```python
from build123d import *

# Parameters (mm, degrees)
CROQUIS1_R              = 9.25
SALIENTE_EXTRUIR1_DEPTH = 9.75
REDONDEO4_R             = 3
REDONDEO5_R             = 2
REDONDEO6_R             = 5


with BuildPart() as part:
    # Croquis1 → Saliente-Extruir1 (new, symmetric)
    with BuildSketch(Plane.XY):
        with BuildLine():
            Line((16.461713879, 5.938179534), (18.205490224, 1.104114294))
            ThreePointArc((18.205490224, 1.104114294), (19.855946903, -1.814596224), (22.378427867, -4.023661212))
            ThreePointArc((22.378427867, -4.023661212), (30.919049272, -8.178302275), (40.105510362, -10.589150466))
            ThreePointArc((40.105510362, -10.589150466), (44.326282594, -12.959198031), (46, -17.50130258))
            Line((46, -17.50130258), (46, -18.509558121))
            Line((46, -18.509558121), (46, -43))
            Line((46, -43), (15, -43))
            Line((15, -43), (12, -18))
            Line((12, -18), (-12, -18))
            Line((-12, -18), (-15, -43))
            Line((-15, -43), (-46, -43))
            Line((-46, -43), (-46, -18.509558121))
            Line((-46, -18.509558121), (-46, -17.50130258))
            ThreePointArc((-46, -17.50130258), (-44.326282594, -12.959198031), (-40.105510362, -10.589150466))
            ThreePointArc((-40.105510362, -10.589150466), (-30.919049272, -8.178302275), (-22.378427867, -4.023661212))
            ThreePointArc((-22.378427867, -4.023661212), (-19.855946903, -1.814596224), (-18.205490224, 1.104114294))
            Line((-18.205490224, 1.104114294), (-16.461713879, 5.938179534))
            ThreePointArc((-16.461713879, 5.938179534), (0, 17.5), (16.461713879, 5.938179534))
        make_face()
        Circle(CROQUIS1_R, mode=Mode.SUBTRACT)
    extrude(amount=SALIENTE_EXTRUIR1_DEPTH, both=True)

    # Redondeo4
    redondeo4_edges = [part.edges().sort_by_distance(p)[0] for p in [
        (12, -18, 0),
        (-12, -18, 0),
    ]]
    fillet(redondeo4_edges, radius=REDONDEO4_R)

    # Redondeo5
    redondeo5_edges = [part.edges().sort_by_distance(p)[0] for p in [
        (-19.855946903, -1.814596224, 9.75),
        (-30.919049272, -8.178302275, 9.75),
        (17.333602052, 3.521146914, -9.75),
        (-44.326282594, -12.959198031, 9.75),
        (19.855946903, -1.814596224, -9.75),
        (30.919049272, -8.178302275, -9.75),
        (44.326282594, -12.959198031, -9.75),
        (46, -30.25065129, -9.75),
        (-46, -30.25065129, 9.75),
        (-13.65855386, -31.821282169, -9.75),
        (-46, -30.25065129, -9.75),
        (-44.326282594, -12.959198031, -9.75),
        (-30.919049272, -8.178302275, -9.75),
        (-19.855946903, -1.814596224, -9.75),
        (-17.333602052, 3.521146914, -9.75),
        (0, 17.5, -9.75),
        (-13.65855386, -31.821282169, 9.75),
        (0, 17.5, 9.75),
        (46, -30.25065129, 9.75),
        (44.326282594, -12.959198031, 9.75),
        (30.919049272, -8.178302275, 9.75),
        (19.855946903, -1.814596224, 9.75),
        (13.65855386, -31.821282169, -9.75),
        (13.65855386, -31.821282169, 9.75),
        (0, -18, -9.75),
        (17.333602052, 3.521146914, 9.75),
        (0, -18, 9.75),
        (11.329418316, -18.755862417, -9.75),
        (11.329418316, -18.755862417, 9.75),
        (-11.329418316, -18.755862417, -9.75),
        (-11.329418316, -18.755862417, 9.75),
        (-17.333602052, 3.521146914, 9.75),
    ]]
    fillet(redondeo5_edges, radius=REDONDEO5_R)

    # Redondeo6
    # the kernel refuses this fillet: 5 mm, written as the material it takes off along each edge
    with BuildSketch(Plane(origin=(56.5, -43, 9.75), x_dir=(0, 1, 0), z_dir=(-1, 0, 0)), Plane(origin=(-4.51434853, -43, 9.75), x_dir=(0, 1, 0), z_dir=(-1, 0, 0)), Plane(origin=(56.5, -43, -9.75), x_dir=(0, 0, 1), z_dir=(-1, 0, 0)), Plane(origin=(-4.51434853, -43, -9.75), x_dir=(0, 0, 1), z_dir=(-1, 0, 0))) as redondeo6_piece_1:
        with BuildLine():
            CenterArc((REDONDEO6_R, REDONDEO6_R), REDONDEO6_R, 180, 90)
            Line((0, REDONDEO6_R), (0, 0))
            Line((0, 0), (REDONDEO6_R, 0))
        make_face()
    extrude(amount=51.98565147, mode=Mode.SUBTRACT)


solid = part.part
```
Verification items for the finished model (mm, model axes). A direction names the side the tool comes from. Coordinates: 2 decimals unless noted, no trailing zeros. Order: outer loops, then holes, each group sorted by start corner. A loop starts at its lowest first (then second) coordinate and runs counter-clockwise, first axis right, second up. Notation, with made-up numbers: (-8.5, 24.25) -> (27.5, 24.25) arc R20 ccw to (27.5, 36.25) -> close; hole circle Ø9 at (14, 76.25). An arc over 180 degrees is marked (long way). Put each result on its own line as item: value. Start each with the question number.
1) Tool access check on faces 4 (the flat face through (46, -30, 0)), 5 (the cylindrical face through (14, -31, -9)), 6 (the cylindrical face through (-0.13, -17.4, 9.18)), 7 (the flat face through (-13.64, -31.66, 0.11)). Record the directions out of +Z, -Z, +X, -X, +Y, -Y that give a thin tool (end or side, any length) a straight path to the whole face; none if there is none.
2) Release check for a two-part mould opening along Y. For faces 1 (the cylindrical face through (-14, -31, -9)), 2 (the cylindrical face through (45.4, -29.92, 9.18)), 3 (the cylindrical face through (-2.01, -9.03, -0.14)) record: pulls with the +Y half, pulls with the -Y half, needs draft (parallel to the pull), parting line crosses it, or undercut.
3) Material ranges on L1, parallel to X at y = -21, z = -3; L2, parallel to Y at x = -2, z = 1.5; L3, parallel to X at y = -22, z = -3.25, recorded low to high.
4) Cross-section at B-B (z = 3). Enter the section's corners in (x, y), plus the area to 3 significant figures.
5) Go/stop test with flat-tipped pins: pin 1 (1.5 mm diameter, centred on x = -10, z = -4.5, fed in from -Y); pin 2 (12 mm diameter, centred on x = -26, y = 11.5, fed in from -Z). Record where each tip stops, or that it passes through.
6) Cross-section at A-A (x = 0). Enter the section's corners in (y, z).
Geometry check:
1. face 4: +Z, -Z, +X, +Y, -Y
1. face 5: -Z, -Y
1. face 6: +Z, -Y
1. face 7: +Z, -Z, -Y
2. face 1: pulls with the -Y half
2. face 2: needs draft
2. face 3: undercut
3. L1: x = -46 to -12.36, 12.36 to 46
3. L2: y = -18 to -9.03, 9.03 to 17.39
3. L3: x = -46 to -12.48, 12.48 to 46
4. outline: (-46, -43) -> (-15, -43) -> (-12.32, -20.64) arc R3 cw to (-9.34, -18) -> (9.34, -18) arc R3 cw to (12.32, -20.64) -> (15, -43) -> (46, -43) -> (46, -17.5) arc R7 ccw to (40.11, -10.59) arc R48.51 cw to (22.38, -4.02) arc R10 cw to (18.21, 1.1) -> (16.46, 5.94) arc R17.5 ccw to (-16.46, 5.94) -> (-18.21, 1.1) arc R10 cw to (-22.38, -4.02) arc R48.51 cw to (-40.11, -10.59) arc R7 ccw to (-46, -17.5) -> close; hole circle Ø18.5 at (0, 0)
4. area: 3,060 mm^2
5. pin 1: stops at y = -18.35
5. pin 2: passes through
6. outline: (-18, -7.75) arc R2 ccw to (-16, -9.75) -> (-9.25, -9.75) -> (-9.25, 9.75) -> (-16, 9.75) arc R2 ccw to (-18, 7.75) -> close; (9.25, -9.75) -> (15.5, -9.75) arc R2 ccw to (17.5, -7.75) -> (17.5, 7.75) arc R2 ccw to (15.5, 9.75) -> (9.25, 9.75) -> close
